Work out the finished part from the listing and answer in its coordinate system (mm). Face numbers are marked on the shaded views. A direction names the side the tool comes from. Coordinates: 2 decimals unless noted, no trailing zeros. Loops run counter-clockwise (first coordinate to the right, second up) from the corner with the lowest first, then second, coordinate; pieces in that order, holes last. Notation, with made-up numbers: (20.25, 39.25) -> (28.25, 39.25) arc R24 ccw to (28.25, 70.25) -> close; hole circle Ø5 at (-17.5, 32.25). An arc over 180 degrees is marked (long way). Use a Markdown table: item, result.
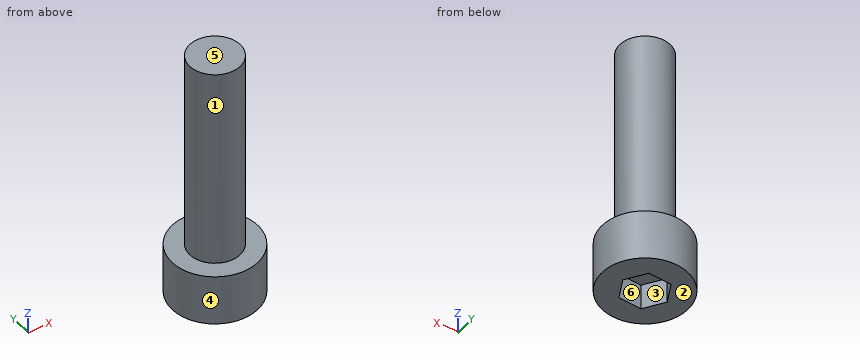
from build123d import *

# Parameters (mm, degrees)
CROQUIS1_R              = 2.5
SALIENTE_EXTRUIR1_DEPTH = 20
CROQUIS2_R              = 4.25
SALIENTE_EXTRUIR2_DEPTH = 5
CORTAR_EXTRUIR1_DEPTH   = 2.5


with BuildPart() as part:
    # Croquis1 → Saliente-Extruir1 (new body)
    with BuildSketch(Plane.XY):
        Circle(CROQUIS1_R)
    extrude(amount=SALIENTE_EXTRUIR1_DEPTH)

    # Croquis2 → Saliente-Extruir2 (add)
    with BuildSketch(Plane(origin=(0, 0, 0), x_dir=(-1, 0, 0), z_dir=(0, 0, -1))):
        Circle(CROQUIS2_R)
    extrude(amount=SALIENTE_EXTRUIR2_DEPTH)

    # Croquis3 → Cortar-Extruir1 (cut)
    with BuildSketch(Plane(origin=(0, 0, -5), x_dir=(-1, 0, 0), z_dir=(0, 0, -1))):
        Polygon((1.267478326, 1.93050046), (-1.038123277, 2.062918659), (-2.305601603, 0.132418199), (-1.267478326, -1.93050046), (1.038123277, -2.062918659), (2.305601603, -0.132418199), align=None)
    extrude(amount=-CORTAR_EXTRUIR1_DEPTH, mode=Mode.SUBTRACT)


solid = part.part
Q1. For the marked faces 1, 2 and 3, determine the directions among +Z, -Z, +X, -X, +Y, -Y from which every point of the face is accessible in a straight line to the end or side of a thin tool.
Solved:
| item | result |
|---|---|
| face 1 | +Z |
| face 2 | -Z, +X, -X, +Y, -Y |
| face 3 | -Z |
Q2. Determine the mould class of the marked faces 4, 5 and 6 for opening direction X: pulls with the +X half, pulls with the -X half, needs draft (parallel to the pull), parting line crosses it, or undercut.
Solved:
| item | result |
|---|---|
| face 4 | parting line crosses it |
| face 5 | needs draft |
| face 6 | undercut |
Q3. Section D-D on z = 11.75 is taken. Determine the outline of the cut face in (x, y), and give its area (3 significant figures).
Solved:
| item | result |
|---|---|
| outline | circle Ø5 at (0, 0) |
| area | 19.6 mm² |
Q4. Section B-B on x = 2 is taken. Determine the outline of the cut face in (y, z), and give its area (3 significant figures).
Solved:
| item | result |
|---|---|
| outline | (-3.75, -5) -> (-0.47, -5) -> (-0.47, -2.5) -> (0.6, -2.5) -> (0.6, -5) -> (3.75, -5) -> (3.75, 0) -> (1.5, 0) -> (1.5, 20) -> (-1.5, 20) -> (-1.5, 0) -> (-3.75, 0) -> close |
| area | 94.8 mm² |
Q5. Section C-C on y = -1.5 is taken. Determine the outline of the cut face in (x, z), and give its area (3 significant figures).
Solved:
| item | result |
|---|---|
| outline | (-3.98, -5) -> (-1.41, -5) -> (-1.41, -2.5) -> (1.48, -2.5) -> (1.48, -5) -> (3.98, -5) -> (3.98, 0) -> (2, 0) -> (2, 20) -> (-2, 20) -> (-2, 0) -> (-3.98, 0) -> close |
| area | 113 mm² |
Q6. Section A-A on z = -3 is taken. Determine the outline of the cut face in (x, y).
Solved:
| item | result |
|---|---|
| outline | circle Ø8.5 at (0, 0); hole (-2.31, -0.13) -> (-1.04, -2.06) -> (1.27, -1.93) -> (2.31, 0.13) -> (1.04, 2.06) -> (-1.27, 1.93) -> close |
Q7. Given pin 1 Ø3 at (x, z) = (2.5, 13.5) entering from -Y; pin 2 Ø1.5 at (x, y) = (0.5, 1) entering from -Z; pin 3 Ø3 at (y, z) = (1.5, 17.5) entering from +X; pin 4 Ø3.5 at (x, y) = (0.5, 0.5) entering from -Z, each flat-ended and moving along its own axis, determine where each tip first touches the part or whether it passes through.
Solved:
| item | result |
|---|---|
| pin 1 | y = -2.29 |
| pin 2 | z = -2.5 |
| pin 3 | x = 2.5 |
| pin 4 | z = -5 |
Q8. Consider line 1 (Z direction, x = -1.25, y = 1.75); line 2 (Z direction, x = -1, y = -2.75); line 3 (X direction, y = 0.75, z = 14). Determine where each line is inside the solid, lowest interval first. Write a range as [from, to].
Solved:
| item | result |
|---|---|
| line 1 | [-2.5, 20] |
| line 2 | [-5, 0] |
| line 3 | [-2.38, 2.38] |
